The model under review builds one solid part; all positions refer to its coordinate system, in mm. A direction names the side the tool comes from. Round coordinates to 2 decimals unless told otherwise and drop trailing zeros. Write each loop counter-clockwise with the first axis right and the second up, starting at its lowest first coordinate (ties: lowest second). Pieces come first, ordered by that corner, then holes. Notation, with made-up numbers: M 35,24.25 L 94,24.25 A20 cw 94,42.25 Z; hole C -22.5,81 d7. An arc over 180 degrees is marked long. One line per item, written item: value. Start each with the question number.
1) Mouldability with a two-part tool opening along X and no side actions: class faces 6 (the face through (-88.9, -1, 25)), 7 (the face through (-101.6, 1, 25)), 8 (the face through (0, 42, 0)) as +X half, -X half, draft (parallel to the pull), parting line (faces both ways), or undercut.
2) For P1, Ø3, axis at x = -25, y = -145, coming from the +Z side; P2, Ø5, axis at x = 24.5, y = -201.5, coming from the -Z side; P3, Ø4, axis at x = -6, y = -91.5, coming from the -Z side, all flat-tipped, find the tip position at first contact; note any pin that passes through.
3) Take a section at A-A, the plane y = -22.5. Write out the cut boundary in (x, z), and give its area (3 significant figures).
4) Wall thickness on probe 1 along Y at (x, z) = (57, 11); probe 2 along X at (y, z) = (-21.5, 20); probe 3 along X at (y, z) = (-239, 55): over which ranges is each line inside the solid? List them lowest first.
5) Tool access review of faces 1 (the face through (0, 42, 50.8)), 2 (the face through (88.9, -1, 25)), 3 (the face through (97.78, -47.18, 25.04)), 4 (the face through (1, 50.8, 25)), 5 (the face through (-2, -283.605, 26)): name each direction out of +Z, -Z, +X, -X, +Y, -Y from which nothing blocks a thin tool from reaching the whole face with its end or side.
from build123d import *

# Parameters (mm, degrees)
F0_W     = 177.8
F0_H     = 76.2
F1_DEPTH = 50.8
F2_W     = 177.8
F2_H     = 50.8
F3_DEPTH = 232.8048453
F3_TAPER = -3


# Not quite as in the source:
# - an extrude ends at something that could not be found from the text; its depth is read off the source's solid


with BuildPart() as f1:
    # F0 (on Top) → F1 (new body)
    with BuildSketch(Plane.XY):
        with BuildLine():
            ThreePointArc((101.6, 38.1), (97.8802561211, 47.0802561211), (88.9, 50.8))
            Line((88.9, 50.8), (-88.9, 50.8))
            ThreePointArc((-88.9, 50.8), (-97.8802561211, 47.0802561211), (-101.6, 38.1))
            Line((-101.6, 38.1), (-101.6, -38.1))
            ThreePointArc((-101.6, -38.1), (-97.8802561211, -47.0802561211), (-88.9, -50.8))
            Line((-88.9, -50.8), (88.9, -50.8))
            ThreePointArc((88.9, -50.8), (97.8802561211, -47.0802561211), (101.6, -38.1))
            Line((101.6, -38.1), (101.6, 38.1))
        make_face()
        Rectangle(F0_W, F0_H, mode=Mode.SUBTRACT)
    extrude(amount=F1_DEPTH)

    # F2 (on face) → F3 (join, through all)
    with BuildSketch(Plane.XZ.offset(50.8)):
        with Locations((0, 25.4)):
            Rectangle(F2_W, F2_H)
    extrude(amount=F3_DEPTH, taper=F3_TAPER)


solid = f1.part
Checked values:
1. face 6: undercut
1. face 7: -X half
1. face 8: draft
2. P1: stops at z = 55.82
2. P2: stops at z = -8.03
2. P3: stops at z = -2.24
3. outline: M -101.6,0 L -88.9,0 L -88.9,50.8 L -101.6,50.8 Z; M 88.9,0 L 101.6,0 L 101.6,50.8 L 88.9,50.8 Z
3. area: 1,290 mm2
4. probe 1: y = -283.6 to -38.1, 38.1 to 50.8
4. probe 2: x = -101.6 to -88.9, 88.9 to 101.6
4. probe 3: x = -98.76 to 98.76
5. face 1: +Z, +X, -X, +Y
5. face 2: +Z, -Z
5. face 3: +Z, -Z, +X
5. face 4: +Z, -Z, +X, -X, +Y
5. face 5: +Z, -Z, +X, -X, -Y
